Source: CAD feature listing. Evaluate the final solid. Frame: model axes, mm. A direction names the side the tool comes from. Round coordinates to 2 decimals unless told otherwise and drop trailing zeros. Order: outer loops, then holes, each group sorted by start corner. A loop starts at its lowest first (then second) coordinate and runs counter-clockwise, first axis right, second up. Notation, with made-up numbers: (13, -11) - (45, -11) arc R21 cw to (45, 13) - close; hole circle Ø6 at (68.25, 71). An arc over 180 degrees is marked (long way). Put each result on its own line as item: value. Start each with the question number.
1) Line query: probe 1 along X at (y, z) = (11.5, -6.25); probe 2 along Z at (x, y) = (-10.25, 2.5); probe 3 along Z at (x, y) = (-4.25, 0.75). Output: solid intervals per line, ascending. Write a range as [from, to].
2) Section D-D on x = 0. Output: boundary loops of the cut face in (y, z), then the cut area to 3 significant figures.
3) Mould query, pull axis X, two halves, no side actions, for faces 1 (the face through (12.1, 7.6, 8.32)), 2 (the face through (-8, 1, -6)), 3 (the face through (-12.7, 7, 0)). Classes: +X half, -X half, draft (parallel to the pull), parting line (faces both ways), or undercut.
4) Access query for faces 4 (the face through (12.1, 7.6, -8.32)), 5 (the face through (0, 3, -6)). Directions: +Z, -Z, +X, -X, +Y, -Y. A direction counts if a zero-diameter tool reaches every point of the face in a straight line with its end or side. Return the directions, or none.
5) Contact query for a flat-ended pin moving along its axis: P1, Ø2, axis at x = -10.16, z = 6.35, coming from the +Y side. Output: stop coordinate, or through.
6) Section B-B on y = 4.5. Output: boundary loops of the cut face in (x, z).
7) Section C-C on x = 10.16. Output: boundary loops of the cut face in (y, z).
8) Section A-A on z = 6.35. Output: boundary loops of the cut face in (x, y).
```python
from build123d import *

# Parameters (mm, degrees)
SKETCH1_W               = 25.4
SKETCH1_H               = 17.78
BOSS_EXTRUDE1_DEPTH     = 15
SKETCH2_W               = 14
SKETCH2_H               = 9
CUT_EXTRUDE1_DEPTH      = 4
SKETCH3_R               = 4
CUT_EXTRUDE2_DEPTH      = 25
SKETCH4_R               = 1.2
CUT_EXTRUDE3_DEPTH      = 25
FILLET1_R               = 2
CHAMFER1_SIZE           = 0.5
SKETCH5_W               = 16
SKETCH5_H               = 2
CUT_EXTRUDE4_DEPTH      = 7
CUT_EXTRUDE4_DEPTH_BACK = 3


with BuildPart() as part:
    # Sketch1 → Boss-Extrude1 (new body)
    with BuildSketch(Plane(origin=(0, 0, 0), x_dir=(1, 0, 0), z_dir=(0, 1, 0))):
        Rectangle(SKETCH1_W, SKETCH1_H)
    extrude(amount=BOSS_EXTRUDE1_DEPTH)

    # Sketch2 → Cut-Extrude1 (cut)
    with BuildSketch(Plane.XZ):
        Rectangle(SKETCH2_W, SKETCH2_H)
    extrude(amount=-CUT_EXTRUDE1_DEPTH, mode=Mode.SUBTRACT)

    # Sketch3 → Cut-Extrude2 (cut)
    with BuildSketch(Plane(origin=(0, 15, 0), x_dir=(1, 0, 0), z_dir=(0, 1, 0))):
        Circle(SKETCH3_R)
    extrude(amount=-CUT_EXTRUDE2_DEPTH, mode=Mode.SUBTRACT)

    # Sketch4 → Cut-Extrude3 (cut)
    with BuildSketch(Plane.XZ):
        with Locations((-10.16, -6.35)):
            Circle(SKETCH4_R)
        with Locations((-10.16, 6.35)):
            Circle(SKETCH4_R)
        with Locations((10.16, 6.35)):
            Circle(SKETCH4_R)
        with Locations((10.16, -6.35)):
            Circle(SKETCH4_R)
    extrude(amount=-CUT_EXTRUDE3_DEPTH, mode=Mode.SUBTRACT)

    # Fillet1
    fillet1_edges = [part.edges().sort_by_distance(p)[0] for p in [
        (-12.7, 7.5, -8.89),
        (12.7, 7.5, -8.89),
        (12.7, 7.5, 8.89),
        (-12.7, 7.5, 8.89),
    ]]
    fillet(fillet1_edges, radius=FILLET1_R)

    # Chamfer1
    chamfer1_edges = [part.edges().sort_by_distance(p)[0] for p in [
        (7, 0, 0),
        (0, 0, 4.5),
        (-7, 0, 0),
        (0, 0, -4.5),
        (8.96, 0, -6.35),
        (8.96, 0, 6.35),
        (-11.36, 0, 6.35),
        (-11.36, 0, -6.35),
    ]]
    chamfer(chamfer1_edges, length=CHAMFER1_SIZE)

    # Sketch5 → Cut-Extrude4 (cut, two sides)
    with BuildSketch(Plane.XZ) as cut_extrude4_sk:
        with Locations((0, -6.39)):
            Rectangle(SKETCH5_W, SKETCH5_H)
    extrude(amount=CUT_EXTRUDE4_DEPTH, mode=Mode.SUBTRACT)
    extrude(cut_extrude4_sk.sketch, amount=-CUT_EXTRUDE4_DEPTH_BACK, mode=Mode.SUBTRACT)


solid = part.part
```
Answer sheet:
1. probe 1: [-12.7, -11.36], [-8.96, 8.96], [11.36, 12.7]
1. probe 2: [-8.89, -7.55], [-5.15, 5.15], [7.55, 8.89]
1. probe 3: [-8.89, -7.39], [-5.39, -4.5], [4.5, 8.89]
2. outline: (0, -8.89) - (15, -8.89) - (15, -4) - (4, -4) - (4, -4.5) - (0.5, -4.5) - (0, -5) - (0, -5.39) - (3, -5.39) - (3, -7.39) - (0, -7.39) - close; (0, 5) - (0.5, 4.5) - (4, 4.5) - (4, 4) - (15, 4) - (15, 8.89) - (0, 8.89) - close
2. area: 136 mm^2
3. face 1: +X half
3. face 2: undercut
3. face 3: -X half
4. face 4: -Z, +X, +Y, -Y
4. face 5: -Y
5. P1: through
6. outline: (-12.7, -6.89) arc R2 ccw to (-10.7, -8.89) - (10.7, -8.89) arc R2 ccw to (12.7, -6.89) - (12.7, 6.89) arc R2 ccw to (10.7, 8.89) - (-10.7, 8.89) arc R2 ccw to (-12.7, 6.89) - close; hole circle Ø2.4 at (-10.16, -6.35); hole circle Ø2.4 at (-10.16, 6.35); hole circle Ø8 at (0, 0); hole circle Ø2.4 at (10.16, -6.35); hole circle Ø2.4 at (10.16, 6.35)
7. outline: (0, -8.89) - (15, -8.89) - (15, -7.55) - (0.5, -7.55) - (0, -8.05) - close; (0, -4.65) - (0.5, -5.15) - (15, -5.15) - (15, 5.15) - (0.5, 5.15) - (0, 4.65) - close; (0, 8.05) - (0.5, 7.55) - (15, 7.55) - (15, 8.89) - (0, 8.89) - close
8. outline: (-12.7, 0) - (-11.86, 0) - (-11.36, 0.5) - (-11.36, 15) - (-12.7, 15) - close; (-8.96, 0.5) - (-8.46, 0) - (8.46, 0) - (8.96, 0.5) - (8.96, 15) - (-8.96, 15) - close; (11.36, 0.5) - (11.86, 0) - (12.7, 0) - (12.7, 15) - (11.36, 15) - close
